The model under review builds one solid part; all positions refer to its coordinate system, in mm. Face numbers are marked on the shaded views. A direction names the side the tool comes from. Round coordinates to 2 decimals unless told otherwise and drop trailing zeros. Write each loop counter-clockwise with the first axis right and the second up, starting at its lowest first coordinate (ties: lowest second). Pieces come first, ordered by that corner, then holes. Notation, with made-up numbers: M -27,45 L 10,45 A26 ccw 10,68 Z; hole C 79.25,50 d9. An arc over 180 degrees is marked long. One line per item, written item: value. Start each with the question number.
1) Take a section at C-C, the plane z = -7. Write out the cut boundary in (x, y), and give its area (3 significant figures).
2) Wall thickness on probe 1 along Y at (x, z) = (-43, -47.5); probe 2 along X at (y, z) = (-8, -77.5); probe 3 along Z at (x, y) = (0.5, 8.5): over which ranges is each line inside the solid? List them lowest first.
3) Tool access review of the marked faces 1, 2 and 3: name each direction out of +Z, -Z, +X, -X, +Y, -Y from which nothing blocks a thin tool from reaching the whole face with its end or side.
4) For P1, Ø12, axis at x = -39, z = -64, coming from the -Y side; P2, Ø8, axis at x = 36, z = -20.5, coming from the +Y side; P3, Ø2.5, axis at x = 12, y = -15, coming from the -Z side; P4, Ø12, axis at y = 0.5, z = -26, coming from the +X side, all flat-tipped, find the tip position at first contact; note any pin that passes through.
5) Take a section at B-B, the plane x = 38.5. Write out the cut boundary in (y, z).
6) Take a section at A-A, the plane x = 0. Write out the cut boundary in (y, z).
7) Mouldability with a two-part tool opening along X and no side actions: class the marked faces 4, 5 and 6 as +X half, -X half, draft (parallel to the pull), parting line (faces both ways), or undercut.
8) Take a section at D-D, the plane x = -13.5. Write out the cut boundary in (y, z).
from build123d import *

# Parameters (mm, degrees)
EXTRUDE_3_DEPTH     = 18
SKETCH_8_W          = 100
SKETCH_8_H          = 106
CUT_EXTRUDE_1_DEPTH = 8
EXTRUDE_5_REACH     = 98.125
CUT_EXTRUDE_2_REACH = 98.125
SKETCH_18_R         = 30


with BuildPart() as part:
    # 草圖7 → 填料-伸長3 (new body)
    with BuildSketch(Plane(origin=(0, 0, 0), x_dir=(1, 0, 0), z_dir=(0, 1, 0))):
        with BuildLine():
            Line((-50, 0), (50, 0))
            Line((50, 0), (50, 68))
            ThreePointArc((50, 68), (0, 118), (-50, 68))
            Line((-50, 68), (-50, 0))
        make_face()
    extrude(amount=-EXTRUDE_3_DEPTH)

    # 草圖8 → 除料-伸長1 (cut)
    with BuildSketch(Plane.XZ.offset(18)):
        with Locations((0, -65)):
            Rectangle(SKETCH_8_W, SKETCH_8_H)
    extrude(amount=-CUT_EXTRUDE_1_DEPTH, mode=Mode.SUBTRACT)

    # 填料-伸長5: up to this face of the body (flat: up to its plane)
    extrude_5_end = Plane(part.part.faces().sort_by_distance((0, -10, -60.288575892))[0])
    # 草圖16 → 填料-伸長5 (add, up to the picked face)
    with BuildSketch(Plane(origin=(0, 29.444863729, -51), x_dir=(1, 0, 0), z_dir=(0, 0.866025403784436, 0.5000000000000044)), mode=Mode.PRIVATE) as extrude_5_sk1:
        with BuildLine():
            Line((-40, -58.889727457), (40, -58.889727457))
            Line((40, -58.889727457), (40, -4.889727457))
            ThreePointArc((40, -4.889727457), (0, 35.110272543), (-40, -4.889727457))
            Line((-40, -4.889727457), (-40, -58.889727457))
        make_face()
    extrude_5_tool1 = split(extrude(extrude_5_sk1.sketch, amount=-EXTRUDE_5_REACH, mode=Mode.PRIVATE), bisect_by=extrude_5_end, keep=Keep.BOTH, mode=Mode.PRIVATE)
    add(extrude_5_tool1.solids().sort_by(Axis((0, 21.58727, -37.390249), (0, -0.866025403784436, -0.5000000000000044)))[0])

    # 除料-伸長2: up to this plane
    cut_extrude_2_end = Plane(origin=(0, -10, 0), z_dir=(0, -1, 0))
    # 草圖18 → 除料-伸長2 (cut, up to the surface)
    with BuildSketch(Plane(origin=(0, 29.444863729, -51), x_dir=(1, 0, 0), z_dir=(0, 0.866025403784436, 0.5000000000000044)), mode=Mode.PRIVATE) as cut_extrude_2_sk1:
        with Locations(Location((0, -4.889727457, 0), (0, 0, 270))):
            Circle(SKETCH_18_R)
    cut_extrude_2_tool1 = split(extrude(cut_extrude_2_sk1.sketch, amount=-CUT_EXTRUDE_2_REACH, mode=Mode.PRIVATE), bisect_by=cut_extrude_2_end, keep=Keep.BOTH, mode=Mode.PRIVATE)
    add(cut_extrude_2_tool1.solids().sort_by_distance((0, 27, -46.765372))[0], mode=Mode.SUBTRACT)


solid = part.part
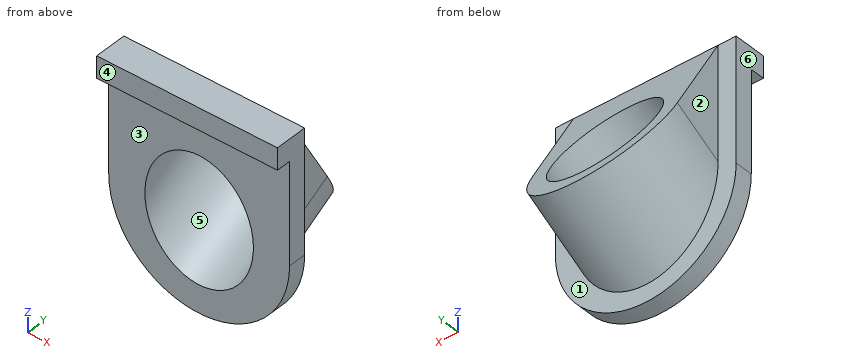
Checked values:
1. outline: M -50,-18 L 50,-18 L 50,0 L 40,0 L 40,4.04 L -40,4.04 L -40,0 L -50,0 Z
1. area: 2,120 mm2
2. probe 1: y = -10 to 0
2. probe 2: x = -49.09 to -28.58, 28.58 to 49.09
2. probe 3: z = -103.63 to -92.08, -22.81 to -14.72
3. face 1: -Z, +Y
3. face 2: +Z, -Z, -X, +Y
3. face 3: -Z, +X, -X, -Y
4. P1: stops at y = -10
4. P2: stops at y = 14.15
4. P3: stops at z = -12
4. P4: stops at x = 50
5. outline: M -18,-12 L -10,-12 L -10,-99.9 L 0,-99.9 L 0,-74.88 L 32.43,-56.16 L 0,0 L -18,0 Z
6. outline: M -18,-12 L -10,-12 L -10,-33.49 L 12,-20.78 L 0,0 L -18,0 Z; M -10,-118 L 0,-118 L 0,-108.54 L 47,-81.41 L 42,-72.75 L -10,-102.77 Z
7. face 4: draft
7. face 5: undercut
7. face 6: -X half
8. outline: M -18,-12 L -10,-12 L -10,-37.19 L 13.6,-23.56 L 0,0 L -18,0 Z; M -10,-116.14 L 0,-116.14 L 0,-105.83 L 45.83,-79.37 L 40.4,-69.97 L -10,-99.06 Z
